from build123d import *

# Parameters (mm, degrees)
BOSS_EXTRUDE1_DEPTH      = 166.889082
BOSS_EXTRUDE1_DEPTH_BACK = 238.865534
SKETCH1_W                = 22
SKETCH1_H                = 100
CAVITY1_START            = -191
CAVITY1_OUTLINE_W        = 40
CAVITY1_OUTLINE_H        = 2
CAVITY1_DEPTH            = 357.889082162


# Read off the part's stored shape, not the designer's step: Cavity1
with BuildPart() as part:
    # Sketch1 → Boss-Extrude1 (new, two sides: drawn at the far end of the back side and taken through both)
    with BuildSketch(Plane(origin=(0, 0, 0), x_dir=(0, 0, -1), z_dir=(1, 0, 0)).offset(-BOSS_EXTRUDE1_DEPTH_BACK)):
        with Locations((1, -190)):
            Rectangle(SKETCH1_W, SKETCH1_H)
    extrude(amount=BOSS_EXTRUDE1_DEPTH + BOSS_EXTRUDE1_DEPTH_BACK)

    # Cavity1 outline → Cavity1 (cut)
    with BuildSketch(Plane.YZ.offset(CAVITY1_START)):
        with Locations((-160, -1)):
            Rectangle(CAVITY1_OUTLINE_W, CAVITY1_OUTLINE_H)
    cavity1 = extrude(amount=CAVITY1_DEPTH, mode=Mode.SUBTRACT)

    # Mirror1: Cavity1 across plane
    add(cavity1.mirror(Plane.ZX.offset(-190)), mode=Mode.SUBTRACT)


solid = part.part
Model file for the job. Use its own axes, mm. A direction names the side the tool comes from. Give positions to 0.01 mm unless a question says otherwise; leave off trailing zeros. Write each loop counter-clockwise with the first axis right and the second up, starting at its lowest first coordinate (ties: lowest second). Pieces come first, ordered by that corner, then holes. Notation, with made-up numbers: (1, 14) - (35, 14) arc R24 cw to (35, 25) - close; hole circle Ø10 at (29, -24.75). An arc over 180 degrees is marked (long way). Answer as CSV lines item,"result".
1. Band-saw the part on B-B (x = -12.5). Write the cut outline in (y, z), and give its area (3 significant figures).
Responses:
outline,"(-240, -12) - (-140, -12) - (-140, -2) - (-180, -2) - (-180, 0) - (-140, 0) - (-140, 10) - (-240, 10) - (-240, 0) - (-200, 0) - (-200, -2) - (-240, -2) - close"
area,"2,040 mm2"
2. 3-axis set-ups, long thin cutter, end or side, ignore diameter. For faces 4 (the face through (-15, -220, 0)), 5 (the face through (-39, -140, 2)), 6 (the face through (-15, -160, 0)): which of +Z, -Z, +X, -X, +Y, -Y reach the whole face in a straight line?
Responses:
face 4,"+X, -Y"
face 5,"+Z, -Z, +X, -X, +Y"
face 6,"+X, +Y"
3. Two-plate mould, pull along Z, no slides. Class faces 1 (the face through (-39, -191, -12)), 2 (the face through (-39, -240, 2)), 3 (the face through (-15, -160, -2)): +Z half, -Z half, draft (parallel to the pull), parting line (faces both ways), or undercut.
Responses:
face 1,"-Z half"
face 2,"draft"
face 3,"undercut"
4. Pin check, flat tips, straight feed: pin 1 (0.6 mm diameter, centred on x = 27, z = -1, fed in from -Y); pin 2 (0.6 mm diameter, centred on y = -163, z = -0.5, fed in from +X). Stop position of each tip, or through.
Responses:
pin 1,"stops at y = -200"
pin 2,"stops at x = -191"
5. Band-saw the part on A-A (y = -227). Write the cut outline in (x, z).
Responses:
outline,"(-238.87, -12) - (166.89, -12) - (166.89, -2) - (-191, -2) - (-191, 0) - (166.89, 0) - (166.89, 10) - (-238.87, 10) - close"
6. Drill centre lines: L1, parallel to Z at x = -35.5, y = -162.5; L2, parallel to X at y = -213, z = -0.75; L3, parallel to Y at x = -17, z = -1.25. Where is each one in solid material? Low to high. Write a range as [from, to].
Responses:
L1,"z = [-12, -2], [0, 10]"
L2,"x = [-238.87, -191]"
L3,"y = [-200, -180]"
